Part model, mm, in its own coordinate system. Face numbers are marked on the shaded views. A direction names the side the tool comes from. Give positions to 0.01 mm unless a question says otherwise; leave off trailing zeros. Write each loop counter-clockwise with the first axis right and the second up, starting at its lowest first coordinate (ties: lowest second). Pieces come first, ordered by that corner, then holes. Notation, with made-up numbers: M 45,-28.5 L 72,-28.5 A22 cw 72,-2.5 Z; hole C 40.5,-9 d2. An arc over 180 degrees is marked long. Answer as CSV lines item,"result". Start each with the question number.
Item 1: Band-saw the part on D-D, the plane x = -6.5. List the corners of the cut face in (y, z).
Item 2: Band-saw the part on A-A, the plane x = 0. List the corners of the cut face in (y, z), then the cut area to 3 significant figures.
Item 3: Band-saw the part on B-B, the plane z = 0.35. List the corners of the cut face in (x, y), then the cut area to 3 significant figures.
Item 4: Wall check: L1, parallel to Y at x = 0, z = 0.6; L2, parallel to Y at x = -5, z = 2.05; L3, parallel to X at y = 0.5, z = 0.55. Give the ranges that are in metal, low to high. Write a range as from..to.
Item 5: Two-plate mould, pull along X, no slides. Class the marked faces 1, 2 and 3: +X half, -X half, draft (parallel to the pull), parting line (faces both ways), or undercut.
Item 6: Pin check, flat tips, straight feed: pin 1 (1.2 mm diameter, centred on y = 11.5, z = 1, fed in from -X); pin 2 (2.5 mm diameter, centred on x = 0, y = 0, fed in from +Z). Stop position of each tip, or through.
Item 7: Band-saw the part on C-C, the plane y = 18. List the corners of the cut face in (x, z), then the cut area to 3 significant figures.
Item 8: 3-axis set-ups, long thin cutter, end or side, ignore diameter. For the marked faces 4, 5 and 6: which of +Z, -Z, +X, -X, +Y, -Y reach the whole face in a straight line?
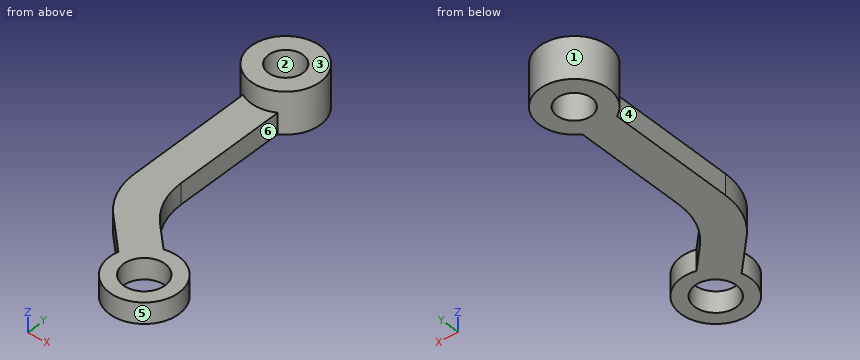
from build123d import *

# Parameters (mm, degrees)
SKETCH1_R           = 1.5
BOSS_EXTRUDE1_DEPTH = 1.5
SKETCH1_3_R         = 2.5
SKETCH1_3_R_2       = 1.25
BOSS_EXTRUDE2_DEPTH = 3


with BuildPart() as part:
    # Sketch1 → Boss-Extrude1 (new body)
    with BuildSketch(Plane.XY):
        with BuildLine():
            Line((-3.75, 7.588834765), (-3.75, 15.834936491))
            ThreePointArc((-3.75, 15.834936491), (-5, 15.5), (-6.25, 15.834936491))
            Line((-6.25, 15.834936491), (-6.25, 6.553300859))
            ThreePointArc((-6.25, 6.553300859), (-5.869397663, 4.639883697), (-4.785533906, 3.017766953))
            Line((-4.785533906, 3.017766953), (-2.414814566, 0.647047613))
            ThreePointArc((-2.414814566, 0.647047613), (1.767766953, -1.767766953), (-0.647047613, 2.414814566))
            Line((-0.647047613, 2.414814566), (-2.285533906, 4.053300859))
            ThreePointArc((-2.285533906, 4.053300859), (-3.369397663, 5.675417603), (-3.75, 7.588834765))
        make_face()
        Circle(SKETCH1_R, mode=Mode.SUBTRACT)
    extrude(amount=BOSS_EXTRUDE1_DEPTH)

    # Sketch1_3 → Boss-Extrude2 (add)
    with BuildSketch(Plane.XY):
        with Locations(Location((-5, 18, 0), (0, 0, 240))):
            Circle(SKETCH1_3_R)
        with Locations((-5, 18)):
            Circle(SKETCH1_3_R_2, mode=Mode.SUBTRACT)
    extrude(amount=BOSS_EXTRUDE2_DEPTH)


solid = part.part
Output:
1,outline,"M 16,0 L 20,0 L 20,3 L 16,3 Z"
2,outline,"M -2.5,0 L -1.5,0 L -1.5,1.5 L -2.5,1.5 Z; M 1.5,0 L 2.5,0 L 2.5,1.5 L 1.5,1.5 Z"
2,area,"3.00 mm²"
3,outline,"M -6.25,6.55 A5 ccw -4.79,3.02 L -2.41,0.65 A2.5 ccw long -0.65,2.41 L -2.29,4.05 A5 cw -3.75,7.59 L -3.75,15.83 A2.5 ccw long -6.25,15.83 Z; hole C -5,18 d2.5; hole C 0,0 d3"
3,area,"65.5 mm²"
4,L1,"-2.5..-1.5, 1.5..2.5"
4,L2,"15.5..16.75, 19.25..20.5"
4,L3,"-2.45..-1.41, 1.41..2.45"
5,face 1,"parting line"
5,face 2,"undercut"
5,face 3,"draft"
6,pin 1,"x = -6.25"
6,pin 2,"through"
7,outline,"M -7.5,0 L -6.25,0 L -6.25,3 L -7.5,3 Z; M -3.75,0 L -2.5,0 L -2.5,3 L -3.75,3 Z"
7,area,"7.50 mm²"
8,face 4,"+Z, -Z, -X, -Y"
8,face 5,"+Z, -Z"
8,face 6,"+Z, -Z, +X"
